CAD build for the part. Positions are in the model's coordinates, mm. A direction names the side the tool comes from. Round coordinates to 2 decimals unless told otherwise and drop trailing zeros. Loops run counter-clockwise (first coordinate to the right, second up) from the corner with the lowest first, then second, coordinate; pieces in that order, holes last.
from build123d import *

# Parameters (mm, degrees)
BOSS_EXTRUDE1_DEPTH = 63.4
BOSS_EXTRUDE2_DEPTH = 2.5
BOSS_EXTRUDE3_DEPTH = 63.4
SKETCH4_R           = 35
CUT_EXTRUDE1_DEPTH  = 152.762941692


with BuildPart() as part:
    # Sketch1 → Boss-Extrude1 (new body)
    with BuildSketch(Plane(origin=(0, 0, 0), x_dir=(1, 0, 0), z_dir=(0, 1, 0))):
        with BuildLine():
            Line((-108.164150322, 11.807033697), (-113.772816425, 5.431031062))
            Line((-113.772816425, 5.431031062), (-110.443441346, 5.431031062))
            Line((-110.443441346, 5.431031062), (-106.2683534, 10.177323898))
            ThreePointArc((-106.2683534, 10.177323898), (3.7316466, 60.67425262), (113.7316466, 10.177323898))
            Line((113.7316466, 10.177323898), (117.906734545, 5.431031062))
            Line((117.906734545, 5.431031062), (121.236109625, 5.431031062))
            Line((121.236109625, 5.431031062), (115.627443521, 11.807033697))
            ThreePointArc((115.627443521, 11.807033697), (3.7316466, 63.17425262), (-108.164150322, 11.807033697))
        make_face()
    extrude(amount=BOSS_EXTRUDE1_DEPTH)

    # Sketch2 → Boss-Extrude2 (add)
    with BuildSketch(Plane(origin=(0, 63.4, 0), x_dir=(1, 0, 0), z_dir=(0, 1, 0))):
        with BuildLine():
            Line((-113.772816425, 5.431031062), (121.236109625, 5.431031062))
            Line((121.236109625, 5.431031062), (115.627443521, 11.807033697))
            ThreePointArc((115.627443521, 11.807033697), (3.7316466, 63.17425262), (-108.164150322, 11.807033697))
            Line((-108.164150322, 11.807033697), (-113.772816425, 5.431031062))
        make_face()
    extrude(amount=BOSS_EXTRUDE2_DEPTH)

    # Sketch3 → Boss-Extrude3 (add)
    with BuildSketch(Plane(origin=(0, 0, 0), x_dir=(1, 0, 0), z_dir=(0, 1, 0))):
        with BuildLine():
            Line((-110.443441346, 5.431031062), (-106.2683534, 10.177323898))
            ThreePointArc((-106.2683534, 10.177323898), (3.7316466, 60.67425262), (113.7316466, 10.177323898))
            Line((113.7316466, 10.177323898), (117.906734545, 5.431031062))
            Line((117.906734545, 5.431031062), (114.515000518, 5.431031062))
            Line((114.515000518, 5.431031062), (111.835849678, 8.547614098))
            ThreePointArc((111.835849678, 8.547614098), (3.7316466, 58.17425262), (-104.372556479, 8.547614098))
            Line((-104.372556479, 8.547614098), (-107.051707318, 5.431031062))
            Line((-107.051707318, 5.431031062), (-110.443441346, 5.431031062))
        make_face()
    extrude(amount=BOSS_EXTRUDE3_DEPTH)

    # Sketch4 → Cut-Extrude1 (cut, through all)
    with BuildSketch(Plane(origin=(0, 65.9, 0), x_dir=(1, 0, 0), z_dir=(0, 1, 0))):
        with Locations((3.7316466, 5.431031062)):
            Circle(SKETCH4_R)
    extrude(amount=-CUT_EXTRUDE1_DEPTH, mode=Mode.SUBTRACT)


solid = part.part
Item 1: Wall check: L1, parallel to Y at x = 102, z = -13; L2, parallel to X at y = 43, z = -26.5; L3, parallel to X at y = 40, z = -23. Give the ranges that are in metal, low to high.
Verdict:
L1: y = 63.4 to 65.9
L2: x = -93.62 to -85.87, 93.33 to 101.09
L3: x = -97.47 to -90.03, 97.49 to 104.93
Item 2: Cut at A-A (z = -34). List the corners of the cut face in (x, y), plus the area to 3 significant figures.
Verdict:
outline: (-84.35, 0) - (-75.69, 0) - (-75.69, 63.4) - (-16.49, 63.4) - (-16.49, 65.9) - (-84.35, 65.9) - close; (23.95, 63.4) - (83.15, 63.4) - (83.15, 0) - (91.81, 0) - (91.81, 65.9) - (23.95, 65.9) - close
area: 1,440 mm2
Item 3: Cut at C-C (z = -45). List the corners of the cut face in (x, y).
Verdict:
outline: (-67.21, 0) - (-56.12, 0) - (-56.12, 63.4) - (63.59, 63.4) - (63.59, 0) - (74.68, 0) - (74.68, 65.9) - (-67.21, 65.9) - close
Item 4: 3-axis set-ups, long thin cutter, end or side, ignore diameter. For faces 1 (the flat face through (4, 0, -60)), 2 (the flat face through (2, 63.4, -44)): which of +Z, -Z, +X, -X, +Y, -Y reach the whole face in a straight line?
Verdict:
face 1: +Z, -Z, +X, -X, -Y
face 2: +Z, -Y
Item 5: Cut at D-D (x = 74). List the corners of the cut face in (y, z), plus the area to 3 significant figures.
Verdict:
outline: (0, -45.37) - (65.9, -45.37) - (65.9, -5.43) - (63.4, -5.43) - (63.4, -39.65) - (0, -39.65) - close
area: 462 mm2
Item 6: Flat gauge pins, fed straight in: P1, Ø10, axis at y = 25.5, z = -48.5, coming from the +X side; P2, Ø12, axis at x = 80, y = 15, coming from the +Z side; P3, Ø5, axis at x = 39, y = 44.5, coming from the -Z side. Where does each tip first touch, or does it go through?
Verdict:
P1: stops at x = 77.35
P2: stops at z = -32.04
P3: stops at z = -59.49
Item 7: Cut at B-B (y = 6.5). List the corners of the cut face in (x, z) (3 decimals).
Verdict:
outline: (-113.773, -5.431) - (-108.164, -11.807) arc R147.558 ccw to (115.627, -11.807) - (121.236, -5.431) - (114.515, -5.431) - (111.836, -8.548) arc R142.558 cw to (-104.373, -8.548) - (-107.052, -5.431) - close
